Autodesk Inventor part; units mm, degrees
ref_plane "YZ Plane" through (0, 0, 0) normal (1, 0, 0) x (0, 1, 0)
ref_plane "XZ Plane" through (0, 0, 0) normal (0, 1, 0) x (-1, 0, 0)
ref_plane "XY Plane" through (0, 0, 0) normal (0, 0, 1) x (1, 0, 0)
sketch "Skizze1" plane through (0, 0, 0) normal (0, 0, 1) x (1, 0, 0)
  circle A0 centre (0, 0) radius 4
  dimension "d0" = 8
extrude "Extrusion1" add sketch "Skizze1" along normal blind 60
fillet "Rundung1" radius 0.5 1 edges at (-4, 0, 0)
sketch "Skizze2" plane through (0, 0, 60) normal (0, 0, 1) x (1, 0, 0)
  circle A0 centre (0, 1.7) radius 0.65
  circle A1 centre (0, -1.7) radius 0.65
  point P0 (0, 0)
  dimension "d4" = 1.3
  dimension "d5" = 1.3
  dimension "d6" = 1.7
  dimension "d7" = 1.7
extrude "Extrusion2" add sketch "Skizze2" along normal blind 10
sketch "Skizze3" plane through (0, 1.7, 70) normal (0, 0, 1) x (1, 0, 0)
  point P0 (0, -1.7)
properties part number "HP_8x60_160W" material "Edelstahl, 440C"
Source: CAD feature listing. Evaluate the final solid. Frame: model axes, mm. A direction names the side the tool comes from. Give positions to 0.01 mm unless a question says otherwise; leave off trailing zeros. Write each loop counter-clockwise with the first axis right and the second up, starting at its lowest first coordinate (ties: lowest second). Pieces come first, ordered by that corner, then holes. Notation, with made-up numbers: (-26.5, -20.5) - (-2.5, -20.5) arc R30 ccw to (-2.5, 13.5) - close; hole circle Ø8 at (-32, -18.75). An arc over 180 degrees is marked (long way). One line per item, written item: value. Start each with the question number.
Q1. Material intervals for probe 1 along Z at (x, y) = (-2.25, 1.75); probe 2 along Y at (x, z) = (-0.5, 67.5); probe 3 along Y at (x, z) = (0.25, 6), sorted ascending. Write a range as from..to.
Q2. First-contact query: pin 1 Ø1 at (x, z) = (2, 27) entering from +Y. Flat tip, straight axial feed; report the tip coordinate or a pass-through.
Q3. Set-up query: faces 4 (the face through (0, -2, 70)), 5 (the face through (-0.085, 1.056, 64.93)). Return all of +Z, -Z, +X, -X, +Y, -Y with unobstructed straight access to the full face (end or side cutting, diameter ignored); none if empty.
Q4. Draft query along Y for faces 1 (the face through (0, 2, 70)), 2 (the face through (-0.867, 3.905, 29.834)), 3 (the face through (-0.141, -1.065, 64.93)). Return one class per face: +Y half, -Y half, draft (parallel to the pull), parting line (faces both ways), or undercut.
Q5. Section query B-B, the plane z = 8.5. Return the cut outline in (x, y), then the cut area to 3 significant figures.
Q6. Section query A-A, the plane x = 0. Return the cut outline in (y, z).
Answer:
1. probe 1: z = 0..60
1. probe 2: y = -2.12..-1.28, 1.28..2.12
1. probe 3: y = -3.99..3.99
2. pin 1: stops at y = 3.71
3. face 4: +Z, +X, -X, +Y, -Y
3. face 5: +Z
4. face 1: draft
4. face 2: parting line
4. face 3: undercut
5. outline: circle Ø8 at (0, 0)
5. area: 50.3 mm2
6. outline: (-4, 0.5) arc R0.5 ccw to (-3.5, 0) - (3.5, 0) arc R0.5 ccw to (4, 0.5) - (4, 60) - (2.35, 60) - (2.35, 70) - (1.05, 70) - (1.05, 60) - (-1.05, 60) - (-1.05, 70) - (-2.35, 70) - (-2.35, 60) - (-4, 60) - close
